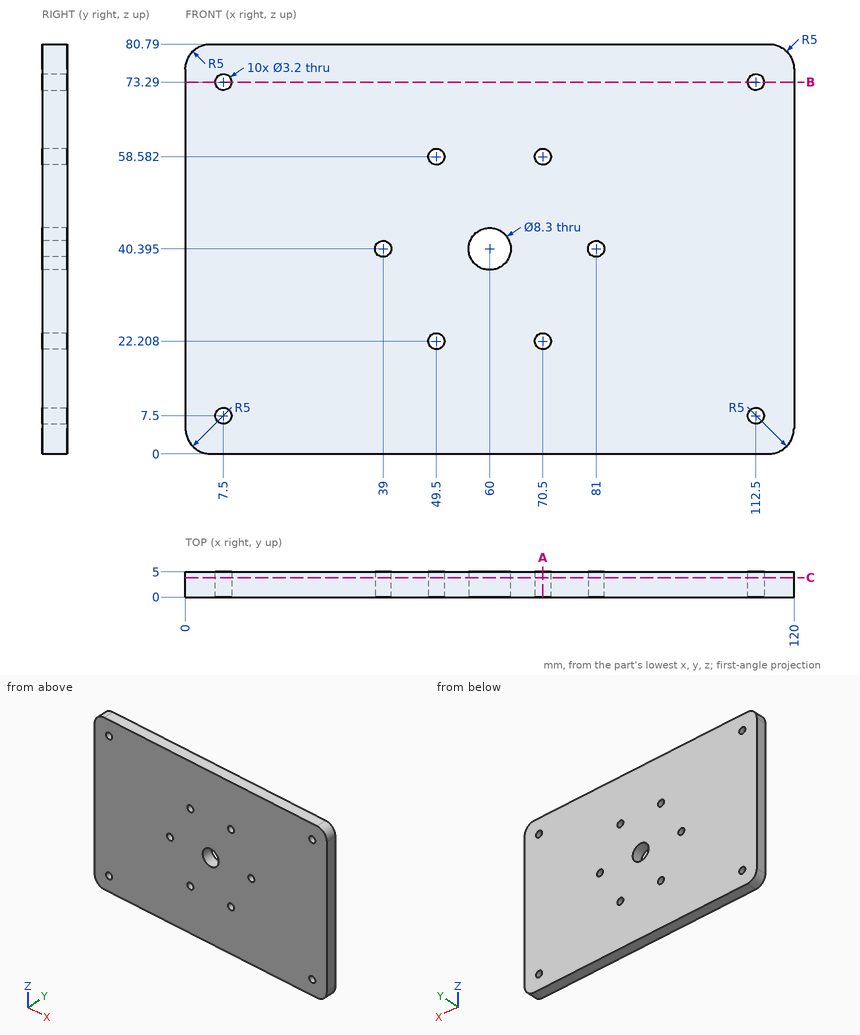
Study the drawing (mm; zero at the part's minimum x, y, z) and answer. Round coordinates to 2 decimals unless told otherwise and drop trailing zeros. Write each loop counter-clockwise with the first axis right and the second up, starting at its lowest first coordinate (ties: lowest second). Pieces come first, ordered by that corner, then holes. Notation, with made-up numbers: (42, 43) -> (84, 43) arc R23 ccw to (84, 59) -> close; hole circle Ø6 at (50.25, 31). An arc over 180 degrees is marked (long way). Answer as CSV lines item,"result". Start each with the question number.
(1) The part is cut by section C-C, the plane y = 3.85. Give the number of separate pieces and of enclosed holes in the cut face, then the cut area to 3 significant figures.
(2) The part is cut by section B-B, the plane z = 73.29. Give the vertices of the cut face in (x, y), then the cut area to 3 significant figures.
(3) Find the intervals of material crossed by probe 1 along X at (y, z) = (1.45, 7.5); probe 2 along Z at (x, y) = (49.5, 2.55); probe 3 along X at (y, z) = (2.85, 7), in increasing order.
(4) Each of these flat-tipped pins is pushed along its axis until it touches: pin 1 (4 mm diameter, centred on x = 81, z = 40.395, fed in from +Y); pin 2 (1.9 mm diameter, centred on x = 49.5, z = 22.21, fed in from +Y). Where does it stop, or does it pass through?
(5) The part is cut by section A-A, the plane x = 70.5. Give the vertices of the cut face in (y, z), then the cut area to 3 significant figures.
Output values:
1,separate pieces,"1"
1,enclosed holes,"11"
1,area,"9,540 mm²"
2,outline,"(0, 0) -> (5.9, 0) -> (5.9, 5) -> (0, 5) -> close; (9.1, 0) -> (110.9, 0) -> (110.9, 5) -> (9.1, 5) -> close; (114.1, 0) -> (120, 0) -> (120, 5) -> (114.1, 5) -> close"
2,area,"568 mm²"
3,probe 1,"x = 0 to 5.9, 9.1 to 110.9, 114.1 to 120"
3,probe 2,"z = 0 to 20.61, 23.81 to 56.98, 60.18 to 80.79"
3,probe 3,"x = 0 to 5.98, 9.02 to 110.98, 114.02 to 120"
4,pin 1,"stops at y = 5"
4,pin 2,"passes through"
5,outline,"(0, 0) -> (5, 0) -> (5, 20.61) -> (0, 20.61) -> close; (0, 23.81) -> (5, 23.81) -> (5, 56.98) -> (0, 56.98) -> close; (0, 60.18) -> (5, 60.18) -> (5, 80.79) -> (0, 80.79) -> close"
5,area,"372 mm²"
